Job drawing, mm, ordinate dimensions from the low corner. One solid piece. A direction names the side the tool comes from. Give positions to 0.01 mm unless a question says otherwise; leave off trailing zeros. Order: outer loops, then holes, each group sorted by start corner. A loop starts at its lowest first (then second) coordinate and runs counter-clockwise, first axis right, second up. Notation, with made-up numbers: M -27.75,29.5 L 5.25,29.5 A27 cw 5.25,46.5 Z; hole C 52.25,69.5 d8. An arc over 180 degrees is marked long. Put each result on its own line as item: value. Start each with the question number.
1) Pin check, flat tips, straight feed: pin 1 (6 mm diameter, centred on y = 13.5, z = 3.5, fed in from +X); pin 2 (8 mm diameter, centred on x = 11, z = 11, fed in from +Y) (3 decimals); pin 3 (8 mm diameter, centred on y = 13, z = 19.5, fed in from -X). Stop position of each tip, or through.
2) Two-plate mould, pull along Z, no slides. Class the marked faces 4, 5 and 6: released by +Z, released by -Z, zero draft, split by the parting line, or undercut.
3) Tool access for the marked faces 1, 2 and 3: list every direction of +Z, -Z, +X, -X, +Y, -Y with a clear straight run to the whole face (end or side of a thin tool).
4) Cut at C-C (z = 19). Write the cut outline in (x, y).
5) Cut at D-D (y = 2.5). Write the cut outline in (x, z), and give its area (3 significant figures).
6) Drill centre lines: line 1 (X direction, y = 10.25, z = 11); line 2 (Z direction, x = 11, y = 8); line 3 (Y direction, x = 17, z = 6.25). Where is each one in solid material? Low to high. Write a range as [from, to].
7) Cut at A-A (x = 11). Write the cut outline in (y, z) (3 decimals), and give its area (3 significant figures).
8) Cut at B-B (z = 11). Write the cut outline in (x, y) (3 decimals).
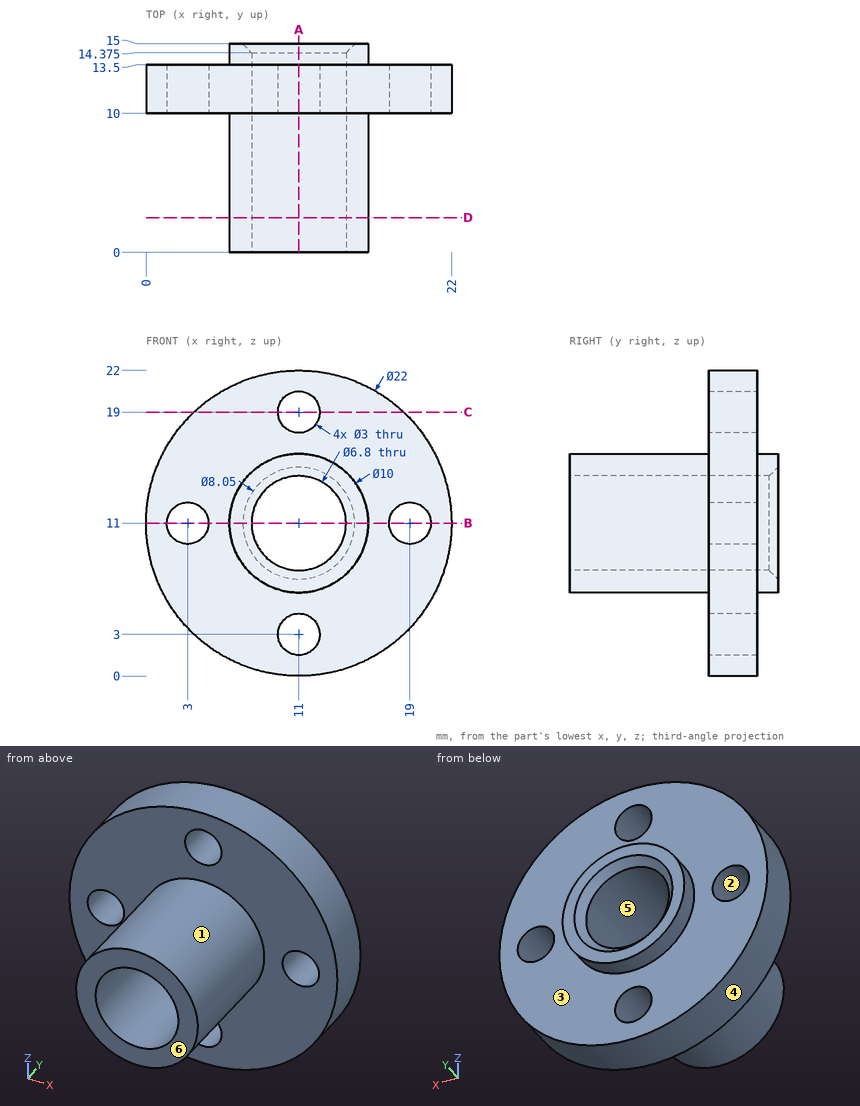
Solution:
1. pin 1: x = 21.04
1. pin 2: y = 14.975
1. pin 3: x = 0.96
2. face 4: split by the parting line
2. face 5: undercut
2. face 6: zero draft
3. face 1: -Y
3. face 2: +Y, -Y
3. face 3: +Y
4. outline: M 3.45,10 L 9.5,10 L 9.5,13.5 L 3.45,13.5 Z; M 12.5,10 L 18.55,10 L 18.55,13.5 L 12.5,13.5 Z
5. outline: C 11,11 d10; hole C 11,11 d6.8
5. area: 42.2 mm²
6. line 1: [0, 1.5], [4.5, 7.6], [14.4, 17.5], [20.5, 22]
6. line 2: [6, 7.6], [14.4, 16]
6. line 3: [10, 13.5]
7. outline: M 0,6 L 10,6 L 10,4.5 L 13.5,4.5 L 13.5,6 L 15,6 L 15,6.975 L 14.375,7.6 L 0,7.6 Z; M 0,14.4 L 14.375,14.4 L 15,15.025 L 15,16 L 13.5,16 L 13.5,17.5 L 10,17.5 L 10,16 L 0,16 Z; M 10,0 L 13.5,0 L 13.5,1.5 L 10,1.5 Z; M 10,20.5 L 13.5,20.5 L 13.5,22 L 10,22 Z
7. area: 68.6 mm²
8. outline: M 0,10 L 1.5,10 L 1.5,13.5 L 0,13.5 Z; M 4.5,10 L 6,10 L 6,0 L 7.6,0 L 7.6,14.375 L 6.975,15 L 6,15 L 6,13.5 L 4.5,13.5 Z; M 14.4,0 L 16,0 L 16,10 L 17.5,10 L 17.5,13.5 L 16,13.5 L 16,15 L 15.025,15 L 14.4,14.375 Z; M 20.5,10 L 22,10 L 22,13.5 L 20.5,13.5 Z
